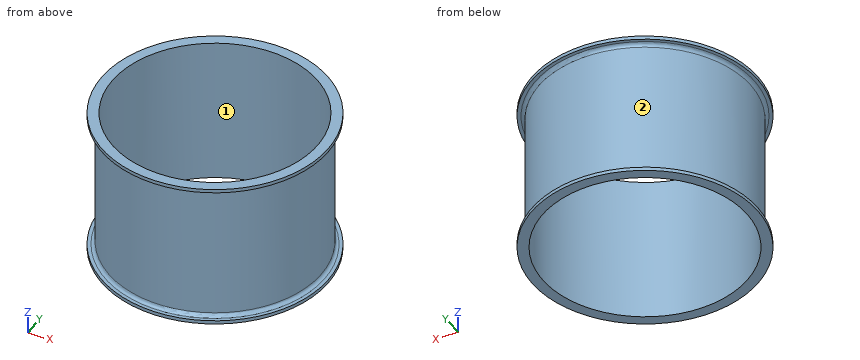
from build123d import *

# Parameters (mm, degrees)
IZIM1_R                     = 160
Y_KSEKLIK_EKSTR_ZYON1_DEPTH = 5
IZIM2_R                     = 150
Y_KSEKLIK_EKSTR_ZYON2_DEPTH = 200
IZIM3_R                     = 160
Y_KSEKLIK_EKSTR_ZYON3_DEPTH = 5
IZIM4_R                     = 145
KES_EKSTR_ZYON1_DEPTH       = 210
RADYUS1_R                   = 5


with BuildPart() as part:
    # Çizim1 → Yükseklik-Ekstrüzyon1 (new body)
    with BuildSketch(Plane.XY):
        Circle(IZIM1_R)
    extrude(amount=Y_KSEKLIK_EKSTR_ZYON1_DEPTH)

    # Çizim2 → Yükseklik-Ekstrüzyon2 (add)
    with BuildSketch(Plane.XY.offset(5)):
        Circle(IZIM2_R)
    extrude(amount=Y_KSEKLIK_EKSTR_ZYON2_DEPTH)

    # Çizim3 → Yükseklik-Ekstrüzyon3 (add)
    with BuildSketch(Plane.XY.offset(205)):
        Circle(IZIM3_R)
    extrude(amount=Y_KSEKLIK_EKSTR_ZYON3_DEPTH)

    # Çizim4 → Kes-Ekstrüzyon1 (cut)
    with BuildSketch(Plane(origin=(0, 0, 0), x_dir=(-1, 0, 0), z_dir=(0, 0, -1))):
        Circle(IZIM4_R)
    extrude(amount=-KES_EKSTR_ZYON1_DEPTH, mode=Mode.SUBTRACT)

    # Radyus1
    radyus1_edges = [part.edges().sort_by_distance(p)[0] for p in [
        (-150, 0, 5),
        (-150, 0, 205),
    ]]
    fillet(radyus1_edges, radius=RADYUS1_R)


solid = part.part
The model under review builds one solid part; all positions refer to its coordinate system, in mm. Face numbers are marked on the shaded views. Coordinates: 2 decimals unless noted, no trailing zeros. Write each loop counter-clockwise with the first axis right and the second up, starting at its lowest first coordinate (ties: lowest second). Pieces come first, ordered by that corner, then holes. Notation, with made-up numbers: (23, -26) - (71, -26) arc R14 ccw to (71, -5) - close; hole circle Ø2 at (11, 83). An arc over 180 degrees is marked (long way). Answer as a JSON object with one key per item and string values. Group by question number.
1. Add section C-C (z = 124). Give the boundary of the cut face in (x, y), plus the area to 3 significant figures.
2. Clearance check with flat-ended pins moving along their axes: pin 1 Ø5 at (x, z) = (51.5, 59.5) entering from +Y; pin 2 Ø3 at (x, z) = (-21, 44.5) entering from +Y; pin 3 Ø1 at (x, z) = (52, 175.5) entering from +Y; pin 4 Ø12 at (x, y) = (118, -124.5) entering from +Z. State where each tip first meets the part, or that it passes through.
3. Add section A-A (x = 0). Give the boundary of the cut face in (y, z), plus the area to 3 significant figures.
4. To check wall thickness, follow probe 1 along Y at (x, z) = (0, 46); probe 2 along Y at (x, z) = (-4.5, 30); probe 3 along X at (y, z) = (78.5, 18). State the ranges of each line that lie inside material, in increasing order.
5. Mouldability with a two-part tool opening along X and no side actions: class the marked faces 1 and 2 as pulls with the +X half, pulls with the -X half, needs draft (parallel to the pull), parting line crosses it, or undercut.
Findings:
{
 "1": {"outline": "circle Ø300 at (0, 0); hole circle Ø290 at (0, 0)", "area": "4,630 mm²"},
 "2": {"pin 1": "y = 141.77", "pin 2": "y = 148.73", "pin 3": "y = 140.88", "pin 4": "through"},
 "3": {"outline": "(-160, 0) - (-145, 0) - (-145, 210) - (-160, 210) - (-160, 205) - (-155, 205) arc R5 cw to (-150, 200) - (-150, 10) arc R5 cw to (-155, 5) - (-160, 5) - close; (145, 0) - (160, 0) - (160, 5) - (155, 5) arc R5 cw to (150, 10) - (150, 200) arc R5 cw to (155, 205) - (160, 205) - (160, 210) - (145, 210) - close", "area": "2,320 mm²"},
 "4": {"probe 1": "-150 to -145, 145 to 150", "probe 2": "-149.93 to -144.93, 144.93 to 149.93", "probe 3": "-127.82 to -121.91, 121.91 to 127.82"},
 "5": {"face 1": "undercut", "face 2": "parting line crosses it"}
}
